Input: dimensioned drawing with shaded views. Units: mm. Origin: part minimum x, y, z. Coordinates: 2 decimals unless noted, no trailing zeros. Write each loop counter-clockwise with the first axis right and the second up, starting at its lowest first coordinate (ties: lowest second). Pieces come first, ordered by that corner, then holes. Notation, with made-up numbers: M 38.25,14 L 47.25,14 A21 cw 47.25,21 Z; hole C -24.5,-19 d1. An arc over 180 degrees is marked long. Use one line per item in the form item = value.
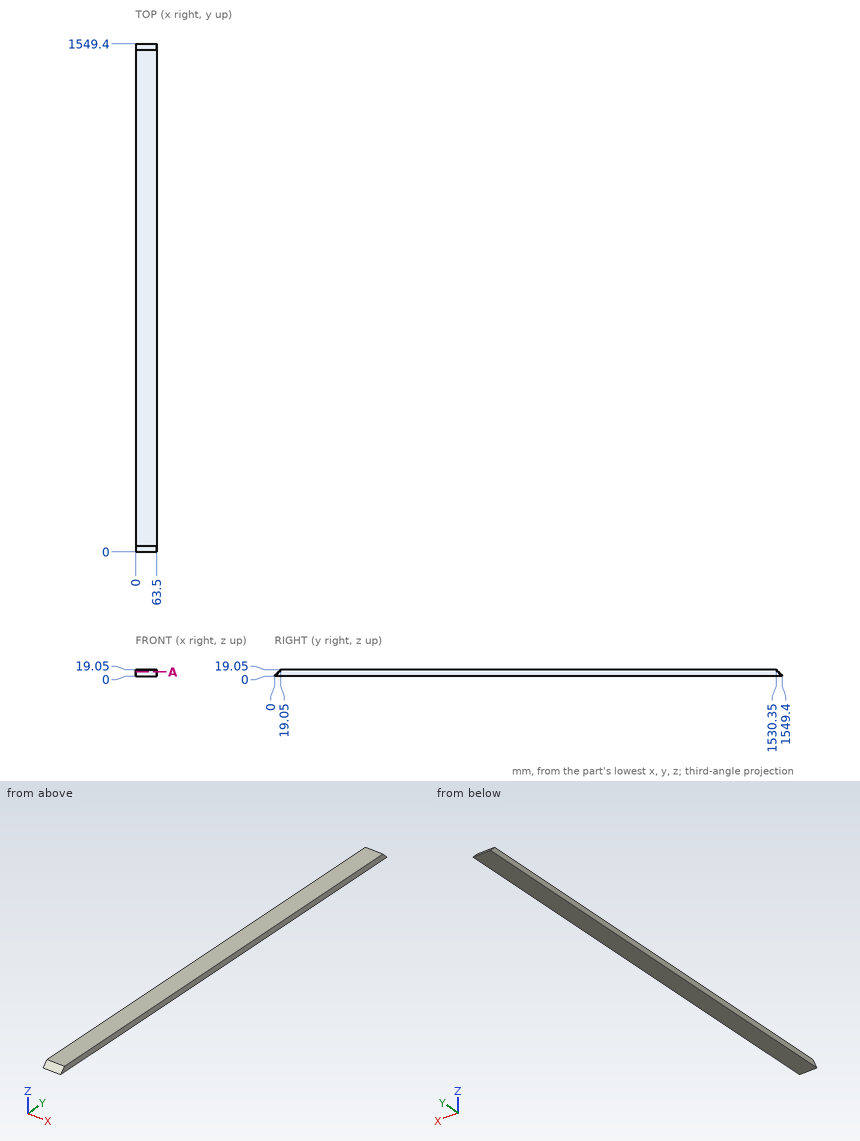
(1) Line query: probe 1 along Y at (x, z) = (46.5, 12); probe 2 along Y at (x, z) = (32, 15.25). Output: solid intervals per line, ascending.
Computed:
probe_1 = 12 to 1537.4
probe_2 = 15.25 to 1534.15
(2) Section query A-A on z = 12.5. Return the cut outline in (x, y).
Computed:
outline = M 0,12.5 L 63.5,12.5 L 63.5,1536.9 L 0,1536.9 Z
(3) First-contact query: pin 1 Ø6 at (x, z) = (12.5, 11.5) entering from -Y; pin 2 Ø6 at (x, z) = (9.5, 12) entering from -Y; pin 3 Ø1 at (x, z) = (24, 14.5) entering from -Y. Flat tips, straight axial feed; report the tip coordinate or a pass-through.
Computed:
pin_1 = 8.5
pin_2 = 9
pin_3 = 14
